```python
from build123d import *

# Parameters (mm, degrees)
SKETCH1_W                                        = 25.4
SKETCH1_H                                        = 25.4
BOSS_EXTRUDE1_DEPTH                              = 8
SKETCH2_W                                        = 5
SKETCH2_H                                        = 25.4
BOSS_EXTRUDE2_DEPTH                              = 5
CBORE_FOR_1_4_SOCKET_HEAD_CAP_SCREW1_D           = 6.7564
CBORE_FOR_1_4_SOCKET_HEAD_CAP_SCREW1_CBORE_D     = 11.1125
CBORE_FOR_1_4_SOCKET_HEAD_CAP_SCREW1_CBORE_DEPTH = 6.35
SKETCH5_W                                        = 15
SKETCH5_H                                        = 3
CUT_EXTRUDE1_DEPTH                               = 36.18983099
SKETCH6_W                                        = 5
SKETCH6_H                                        = 25.4
BOSS_EXTRUDE3_DEPTH                              = 5
SKETCH7_W                                        = 15
SKETCH7_H                                        = 3
CUT_EXTRUDE2_DEPTH                               = 38.327258205
FILLET1_R                                        = 2


with BuildPart() as part:
    # Sketch1 → Boss-Extrude1 (new body)
    with BuildSketch(Plane(origin=(0, 0, 0), x_dir=(1, 0, 0), z_dir=(0, 1, 0))):
        with Locations((2.028136882, -7.895247148)):
            Rectangle(SKETCH1_W, SKETCH1_H)
    extrude(amount=BOSS_EXTRUDE1_DEPTH)

    # Sketch2 → Boss-Extrude2 (add)
    with BuildSketch(Plane(origin=(0, 8, 0), x_dir=(1, 0, 0), z_dir=(0, 1, 0))):
        with Locations((-8.171863118, -7.895247148)):
            Rectangle(SKETCH2_W, SKETCH2_H)
        with Locations((12.228136882, -7.895247148)):
            Rectangle(SKETCH2_W, SKETCH2_H)
    extrude(amount=BOSS_EXTRUDE2_DEPTH)

    # CBORE for 1/4 Socket Head Cap Screw1 (through all)
    with Locations(Plane(origin=(0, 8, 0), x_dir=(1, 0, 0), z_dir=(0, 1, 0))):
        with Locations((22.31346114, -3.943712885), (2.028136882, -7.895247148)):
            CounterBoreHole(CBORE_FOR_1_4_SOCKET_HEAD_CAP_SCREW1_D / 2, CBORE_FOR_1_4_SOCKET_HEAD_CAP_SCREW1_CBORE_D / 2, CBORE_FOR_1_4_SOCKET_HEAD_CAP_SCREW1_CBORE_DEPTH)

    # Sketch5 → Cut-Extrude1 (cut, through all)
    with BuildSketch(Plane.ZY.offset(10.671863118)):
        with Locations((7.895247148, 10)):
            Rectangle(SKETCH5_W, SKETCH5_H)
    extrude(amount=-CUT_EXTRUDE1_DEPTH, mode=Mode.SUBTRACT)

    # Sketch6 → Boss-Extrude3 (add)
    with BuildSketch(Plane(origin=(0, 13, 0), x_dir=(1, 0, 0), z_dir=(0, 1, 0))):
        with Locations((-8.171863118, -7.895247148)):
            Rectangle(SKETCH6_W, SKETCH6_H)
    extrude(amount=BOSS_EXTRUDE3_DEPTH)

    # Sketch7 → Cut-Extrude2 (cut, through all)
    with BuildSketch(Plane.ZY.offset(10.671863118)):
        with Locations((7.895247148, 15)):
            Rectangle(SKETCH7_W, SKETCH7_H)
    extrude(amount=-CUT_EXTRUDE2_DEPTH, mode=Mode.SUBTRACT)

    # Fillet1
    fillet1_edges = [part.edges().sort_by_distance(p)[0] for p in [
        (12.228136882, 13, -4.804752852),
        (12.228136882, 13, 20.595247148),
        (-8.171863118, 18, -4.804752852),
        (-8.171863118, 18, 20.595247148),
    ]]
    fillet(fillet1_edges, radius=FILLET1_R)


solid = part.part
```
Model file for the job. Use its own axes, mm. A direction names the side the tool comes from. Give positions to 0.01 mm unless a question says otherwise; leave off trailing zeros. Write each loop counter-clockwise with the first axis right and the second up, starting at its lowest first coordinate (ties: lowest second). Pieces come first, ordered by that corner, then holes. Notation, with made-up numbers: M -8,38.5 L -1,38.5 A13 ccw -1,48.5 Z; hole C 4.25,76 d5. An arc over 180 degrees is marked long. Use a Markdown table: item, result.
1) Cut at B-B (z = 1.5). List the corners of the cut face in (x, y), and give its area (3 significant figures).
Responses:
| item | result |
|---|---|
| outline | M -10.67,0 L 14.73,0 L 14.73,8.5 L 9.73,8.5 L 9.73,8 L -5.67,8 L -5.67,8.5 L -10.67,8.5 Z; M -10.67,11.5 L -5.67,11.5 L -5.67,13.5 L -10.67,13.5 Z; M -10.67,16.5 L -5.67,16.5 L -5.67,18 L -10.67,18 Z; M 9.73,11.5 L 14.73,11.5 L 14.73,13 L 9.73,13 Z |
| area | 233 mm2 |
2) Pin check, flat tips, straight feed: pin 1 (8 mm diameter, centred on x = 8.5, y = 16, fed in from +Z); pin 2 (6 mm diameter, centred on y = 9.5, z = 11.5, fed in from +X); pin 3 (2.5 mm diameter, centred on x = 13.5, z = 12.5, fed in from +Y); pin 4 (5 mm diameter, centred on x = 5, y = 11.5, fed in from -Z). Stop position of each tip, or through.
Responses:
| item | result |
|---|---|
| pin 1 | stops at z = 20.2 |
| pin 2 | stops at x = 14.73 |
| pin 3 | stops at y = 13 |
| pin 4 | passes through |
3) Tool access for faces 1 (the flat face through (9.728, 12, 8)), 2 (the cylindrical face through (12.263, 12.399, 20.025)), 3 (the flat face through (12, 13, 8)), 4 (the flat face through (-8, 10, 0.395)), 5 (the cylindrical face through (12.263, 12.399, -4.234)): list every direction of +Z, -Z, +X, -X, +Y, -Y with a clear straight run to the whole face (end or side of a thin tool).
Responses:
| item | result |
|---|---|
| face 1 | +Z, -Z, +Y |
| face 2 | +Z, +X, +Y |
| face 3 | +Z, -Z, +X, +Y |
| face 4 | +X, -X |
| face 5 | -Z, +X, +Y |
4) Cut at C-C (y = 15.5). List the corners of the cut face in (x, z).
Responses:
| item | result |
|---|---|
| outline | M -10.67,-4.8 L -5.67,-4.8 L -5.67,0.4 L -10.67,0.4 Z; M -10.67,15.4 L -5.67,15.4 L -5.67,20.6 L -10.67,20.6 Z |
5) Pull direction Y, two halves, no side cores. Call faces 6 (the flat face through (2, 8, 2)), 7 (the flat face through (2, 6, 20.595)), 8 (the flat face through (12, 10, 0.395)): +Y half, -Y half, draft (parallel to the pull), parting line (faces both ways), or undercut.
Responses:
| item | result |
|---|---|
| face 6 | +Y half |
| face 7 | draft |
| face 8 | undercut |
6) Cut at D-D (x = -8.75). List the corners of the cut face in (y, z).
Responses:
| item | result |
|---|---|
| outline | M 0,-4.8 L 16,-4.8 A2 ccw 18,-2.8 L 18,18.6 A2 ccw 16,20.6 L 0,20.6 Z; hole M 8.5,0.4 L 11.5,0.4 L 11.5,15.4 L 8.5,15.4 Z; hole M 13.5,0.4 L 16.5,0.4 L 16.5,15.4 L 13.5,15.4 Z |
7) Drill centre lines: line 1 (Y direction, x = -6.5, z = 11.5); line 2 (X direction, y = 12, z = 0); line 3 (X direction, y = 16.75, z = 6.25). Where is each one in solid material? Low to high. Write a range as from..to.
Responses:
| item | result |
|---|---|
| line 1 | y = 0..8.5, 11.5..13.5, 16.5..18 |
| line 2 | x = -10.67..-5.67, 9.73..14.73 |
| line 3 | x = -10.67..-5.67 |
8) Cut at A-A (y = 10). List the corners of the cut face in (x, z).
Responses:
| item | result |
|---|---|
| outline | M -10.67,-4.8 L -5.67,-4.8 L -5.67,0.4 L -10.67,0.4 Z; M -10.67,15.4 L -5.67,15.4 L -5.67,20.6 L -10.67,20.6 Z; M 9.73,-4.8 L 14.73,-4.8 L 14.73,0.4 L 9.73,0.4 Z; M 9.73,15.4 L 14.73,15.4 L 14.73,20.6 L 9.73,20.6 Z |
